For this review, take the finished solid that the model builds, in its own axes (mm). Face numbers are marked on the shaded views. Give positions to 0.01 mm unless a question says otherwise; leave off trailing zeros. Order: outer loops, then holes, each group sorted by start corner. A loop starts at its lowest first (then second) coordinate and runs counter-clockwise, first axis right, second up. Notation, with made-up numbers: (-28, 21.5) -> (-1, 21.5) arc R25 cw to (-1, 45.5) -> close; hole circle Ø5 at (81.25, 26). An arc over 180 degrees is marked (long way). Use CSV: the item, a comma, the result in double quotes. Start each with the question number.
```python
from build123d import *

# Parameters (mm, degrees)
F0_R     = 1.5
F1_DEPTH = 3


with BuildPart() as f1:
    # F0 (on Top) → F1 (new body)
    with BuildSketch(Plane.XY):
        Polygon((-3.5, 2.020726), (-3.5, -2.020726), (0, -4.041452), (3.5, -2.020726), (3.5, 2.020726), (0, 4.041452), align=None)
        Circle(F0_R, mode=Mode.SUBTRACT)
    extrude(amount=F1_DEPTH)


solid = f1.part
```
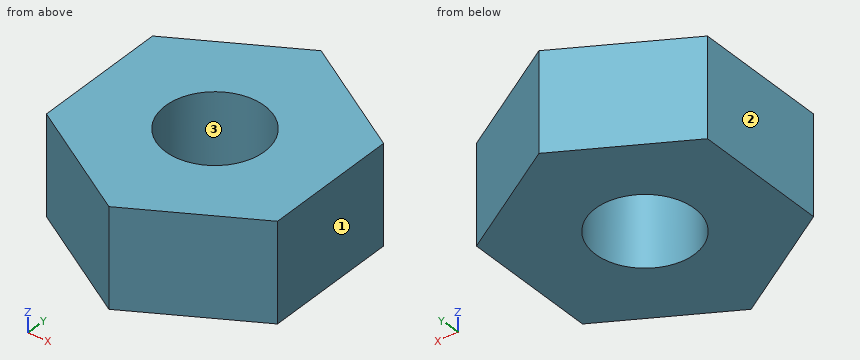
1. Draft analysis for pull direction X (two halves, no side actions). For the marked faces 1, 2 and 3, state which applies: +X half, -X half, draft (parallel to the pull), parting line (faces both ways), or undercut.
2. Consider section D-D (y = 3.5). State the section outline as (x, z) points, plus the area to 3 significant figures.
3. Consider section B-B (x = 0.25). State the section outline as (y, z) points, plus the area to 3 significant figures.
4. Consider section C-C (z = 1.3). State the section outline as (x, y) points.
5. Clearance check with a flat-ended pin moving along its axis: P1, Ø1, axis at x = 2, z = 2.5, coming from the +Y side. State where the tip first meets the part, or that it passes through.
6. Consider section A-A (y = 0). State the section outline as (x, z) points, plus the area to 3 significant figures.
7. To check wall thickness, follow L1, parallel to X at y = 0.75, z = 1.7; L2, parallel to Y at x = 1, z = 0.5; L3, parallel to Y at x = -0.25, z = 1.3. State the ranges of each line that lie inside material, in increasing order. Write a range as [from, to].
Answer list:
1,face 1,"+X half"
1,face 2,"-X half"
1,face 3,"undercut"
2,outline,"(-0.94, 0) -> (0.94, 0) -> (0.94, 3) -> (-0.94, 3) -> close"
2,area,"5.63 mm2"
3,outline,"(-3.9, 0) -> (-1.48, 0) -> (-1.48, 3) -> (-3.9, 3) -> close; (1.48, 0) -> (3.9, 0) -> (3.9, 3) -> (1.48, 3) -> close"
3,area,"14.5 mm2"
4,outline,"(-3.5, -2.02) -> (0, -4.04) -> (3.5, -2.02) -> (3.5, 2.02) -> (0, 4.04) -> (-3.5, 2.02) -> close; hole circle Ø3 at (0, 0)"
5,P1,"y = 3.18"
6,outline,"(-3.5, 0) -> (-1.5, 0) -> (-1.5, 3) -> (-3.5, 3) -> close; (1.5, 0) -> (3.5, 0) -> (3.5, 3) -> (1.5, 3) -> close"
6,area,"12.0 mm2"
7,L1,"[-3.5, -1.3], [1.3, 3.5]"
7,L2,"[-3.46, -1.12], [1.12, 3.46]"
7,L3,"[-3.9, -1.48], [1.48, 3.9]"
